from build123d import *

# Parameters (mm, degrees)
SKETCH1_W           = 56
SKETCH1_H           = 34
SKETCH1_W_2         = 52
SKETCH1_H_2         = 30
BOSS_EXTRUDE1_DEPTH = 1.5
SKETCH1_3_W         = 56
SKETCH1_3_H         = 34
SKETCH1_3_W_2       = 52
SKETCH1_3_H_2       = 30
BOSS_EXTRUDE2_DEPTH = 3
SKETCH2_W           = 53.6
SKETCH2_H           = 31.6
SKETCH2_W_2         = 52
SKETCH2_H_2         = 30
BOSS_EXTRUDE3_DEPTH = 2.3
SKETCH3_W           = 1.2
SKETCH3_H           = 3.75
CUT_EXTRUDE1_DEPTH  = 1
BOSS_EXTRUDE4_START = 13.5
SKETCH4_R           = 0.6
BOSS_EXTRUDE4_DEPTH = 6
FILLET1_R           = 1
FILLET2_R           = 0.8
CUT_EXTRUDE2_DEPTH  = 34.182676203
CUT_EXTRUDE4_DEPTH  = 34.182676203


with BuildPart() as part:
    # Sketch1 → Boss-Extrude1 (new body)
    # profile 1 of 2: a face of its own
    with BuildSketch(Plane(origin=(0, 0, 0), x_dir=(1, 0, 0), z_dir=(0, 1, 0))):
        Rectangle(SKETCH1_W, SKETCH1_H)
        Rectangle(SKETCH1_W_2, SKETCH1_H_2, mode=Mode.SUBTRACT)
    # profile 2 of 2: a face of its own
    with BuildSketch(Plane(origin=(0, 0, 0), x_dir=(1, 0, 0), z_dir=(0, 1, 0))):
        Rectangle(SKETCH1_W_2, SKETCH1_H_2)
    extrude(amount=BOSS_EXTRUDE1_DEPTH)

    # Sketch1_3 → Boss-Extrude2 (add)
    with BuildSketch(Plane(origin=(0, 0, 0), x_dir=(1, 0, 0), z_dir=(0, 1, 0))):
        Rectangle(SKETCH1_3_W, SKETCH1_3_H)
        Rectangle(SKETCH1_3_W_2, SKETCH1_3_H_2, mode=Mode.SUBTRACT)
    extrude(amount=BOSS_EXTRUDE2_DEPTH)

    # Sketch2 → Boss-Extrude3 (add)
    with BuildSketch(Plane(origin=(0, 3, 0), x_dir=(1, 0, 0), z_dir=(0, 1, 0))):
        Rectangle(SKETCH2_W, SKETCH2_H)
        Rectangle(SKETCH2_W_2, SKETCH2_H_2, mode=Mode.SUBTRACT)
    extrude(amount=BOSS_EXTRUDE3_DEPTH)

    # Sketch3 → Cut-Extrude1 (cut)
    with BuildSketch(Plane(origin=(0, 3, 0), x_dir=(1, 0, 0), z_dir=(0, 1, 0))):
        with Locations((-27.4, -8.375)):
            Rectangle(SKETCH3_W, SKETCH3_H)
        with Locations((-27.4, 8.375)):
            Rectangle(SKETCH3_W, SKETCH3_H)
    extrude(amount=-CUT_EXTRUDE1_DEPTH, mode=Mode.SUBTRACT)

    # Sketch4 → Boss-Extrude4 (add)
    with BuildSketch(Plane(origin=(0, 0, 0), x_dir=(0, 0, -1), z_dir=(1, 0, 0)).offset(BOSS_EXTRUDE4_START)):
        with Locations((15.8, 4.7)):
            Circle(SKETCH4_R)
        with Locations((-15.8, 4.7)):
            Circle(SKETCH4_R)
    boss_extrude4 = extrude(amount=BOSS_EXTRUDE4_DEPTH)

    # Mirror1: Boss-Extrude4 across plane
    add(boss_extrude4.mirror(Plane(origin=(0, 0, 0), x_dir=(0, 0, 1), z_dir=(1, 0, 0))))

    # Fillet1
    fillet1_edges = [part.edges().sort_by_distance(p)[0] for p in [
        (0, 0, -17),
        (28, 0, 0),
        (0, 0, 17),
        (-28, 0, 0),
        (-28, 1.5, -17),
        (28, 1.5, -17),
        (28, 1.5, 17),
        (-28, 1.5, 17),
    ]]
    fillet(fillet1_edges, radius=FILLET1_R)

    # Fillet2
    fillet2_edges = [part.edges().sort_by_distance(p)[0] for p in [
        (-26.8, 4.15, -15.8),
        (-26.8, 4.15, 15.8),
        (26.8, 4.15, 15.8),
        (26.8, 4.15, -15.8),
    ]]
    fillet(fillet2_edges, radius=FILLET2_R)

    # Sketch5 → Cut-Extrude2 (cut, through all)
    with BuildSketch(Plane(origin=(0, 0, 0), x_dir=(0, 0, -1), z_dir=(1, 0, 0))):
        with BuildLine():
            Line((-4.5, 9.622902271), (4.5, 9.622902271))
            Line((4.5, 9.622902271), (4.5, 4.9))
            ThreePointArc((4.5, 4.9), (3.914213562, 3.485786438), (2.5, 2.9))
            Line((2.5, 2.9), (-2.5, 2.9))
            ThreePointArc((-2.5, 2.9), (-3.914213562, 3.485786438), (-4.5, 4.9))
            Line((-4.5, 4.9), (-4.5, 9.622902271))
        make_face()
    extrude(amount=-CUT_EXTRUDE2_DEPTH, mode=Mode.SUBTRACT)

    # Sketch7 → Cut-Extrude4 (cut, through all)
    with BuildSketch(Plane.XZ):
        with BuildLine():
            Line((32.037949749, -5.25), (17, -5.25))
            ThreePointArc((17, -5.25), (16.292893219, -4.957106781), (16, -4.25))
            Line((16, -4.25), (16, 4.25))
            ThreePointArc((16, 4.25), (16.292893219, 4.957106781), (17, 5.25))
            Line((17, 5.25), (32.037949749, 5.25))
            Line((32.037949749, 5.25), (32.037949749, -5.25))
        make_face()
    extrude(amount=-CUT_EXTRUDE4_DEPTH, mode=Mode.SUBTRACT)


solid = part.part
Source: CAD feature listing. Evaluate the final solid. Frame: model axes, mm. A direction names the side the tool comes from. Round coordinates to 2 decimals unless told otherwise and drop trailing zeros. Write each loop counter-clockwise with the first axis right and the second up, starting at its lowest first coordinate (ties: lowest second). Pieces come first, ordered by that corner, then holes. Notation, with made-up numbers: M 80,-33 L 90,-33 A22 ccw 90,-21 Z; hole C 68.5,87 d10. An arc over 180 degrees is marked long. One line per item, written item: value. Start each with the question number.
Item 1: Set-up query: faces 4 (the flat face through (24, 1, 5.25)), 5 (the flat face through (-27.4, 2.5, -10.25)), 6 (the flat face through (-27, 2.9, 0)), 7 (the flat face through (26.8, 4, 10)). Return all of +Z, -Z, +X, -X, +Y, -Y with unobstructed straight access to the full face (end or side cutting, diameter ignored); none if empty.
Item 2: Section query D-D (x = -3). Return the cut outline in (y, z), plus the area to 3 significant figures.
Item 3: Pin query (flat end, axial travel): pin 1 (13 mm diameter, centred on x = 9, z = 12.5, fed in from +Y); pin 2 (0.6 mm diameter, centred on x = -26.5, z = 0.5, fed in from +Y); pin 3 (0.8 mm diameter, centred on x = -27.5, y = 2.5, fed in from -Z) (3 decimals); pin 4 (0.7 mm diameter, centred on y = 4, z = -11, fed in from +X). Return the tip coordinate at first contact, or that it passes through.
Item 4: Section query A-A (x = -17.5). Return the cut outline in (y, z), plus the area to 3 significant figures.
Item 5: Section query C-C (z = -7.5). Return the cut outline in (x, y).
Item 6: Mould query, pull axis X, two halves, no side actions, for faces 1 (the cylindrical face through (-27.699, 0.285, -0.224)), 2 (the flat face through (-27, 3, 5)), 3 (the flat face through (26, 3, -10)). Classes: pulls with the +X half, pulls with the -X half, needs draft (parallel to the pull), parting line crosses it, or undercut.
Item 7: Ray query, L1, parallel to Z at x = 21, y = 0.85; L2, parallel to Z at x = -18.5, y = 3.85; L3, parallel to X at y = 1.2, z = 3. Return the intervals inside material, ascending. Write a range as from..to.
Item 8: Section query B-B (z = -1). Return the cut outline in (x, y).
Result set:
1. face 4: +X, +Y, -Y
1. face 5: -X, +Y
1. face 6: +X, -X, +Y
1. face 7: +Z, -Z, +X, +Y
2. outline: M 0,-16 A1 ccw 1,-17 L 3,-17 L 3,-15.8 L 5.3,-15.8 L 5.3,-15 L 1.5,-15 L 1.5,15 L 5.3,15 L 5.3,15.8 L 3,15.8 L 3,17 L 1,17 A1 ccw 0,16 Z
2. area: 60.3 mm²
3. pin 1: stops at y = 5.3
3. pin 2: stops at y = 2.9
3. pin 3: stops at z = -16.995
3. pin 4: stops at x = 26.8
4. outline: M 0,-16 A1 ccw 1,-17 L 3,-17 L 3,-15.8 L 4.1,-15.8 A0.6 ccw 5.3,-15.8 L 5.3,-15 L 1.5,-15 L 1.5,15 L 5.3,15 L 5.3,15.8 A0.6 ccw 4.1,15.8 L 3,15.8 L 3,17 L 1,17 A1 ccw 0,16 Z
4. area: 61.4 mm²
5. outline: M -28,1 A1 ccw -27,0 L 27,0 A1 ccw 28,1 L 28,3 L 26.8,3 L 26.8,5.3 L 26,5.3 L 26,1.5 L -26,1.5 L -26,5.3 L -26.8,5.3 L -26.8,2 L -28,2 Z
6. face 1: pulls with the -X half
6. face 2: needs draft
6. face 3: undercut
7. L1: z = -16.99..-5.25, 5.25..16.99
7. L2: z = -15.8..-15, 15..15.8
7. L3: x = -28..16
8. outline: M -28,1 A1 ccw -27,0 L 16,0 L 16,1.5 L -26,1.5 L -26,2.9 L -28,2.9 Z
